Part print with two shaded views. Sizes in mm from the minimum x, y, z corner. A direction names the side the tool comes from. Round coordinates to 2 decimals unless told otherwise and drop trailing zeros. Loops run counter-clockwise (first coordinate to the right, second up) from the corner with the lowest first, then second, coordinate; pieces in that order, holes last. Notation, with made-up numbers: M -39.5,-1.5 L 8.5,-1.5 A11 ccw 8.5,17.5 Z; hole C 76.5,56.5 d1. An arc over 180 degrees is marked long. Use a Markdown table: item, result. Add a question column.
Item 1: Saw through at B-B on z = 45. Write the cut outline in (x, y), then the cut area to 3 significant figures.
Item 2: Tool access for the marked faces 1 and 2: list every direction of +Z, -Z, +X, -X, +Y, -Y with a clear straight run to the whole face (end or side of a thin tool).
Item 3: Saw through at C-C on y = 25. Write the cut outline in (x, z), then the cut area to 3 significant figures.
Item 4: Pin check, flat tips, straight feed: P1, Ø1, axis at x = 143, z = 96.5, coming from the +Y side; P2, Ø4, axis at y = 72, z = 77.5, coming from the -X side. Stop position of each tip, or through.
Item 5: Two-plate mould, pull along Z, no slides. Class the marked faces 3, 4, 5 and 6: +Z half, -Z half, draft (parallel to the pull), parting line (faces both ways), or undercut.
Item 6: Saw through at A-A on y = 7. Write the cut outline in (x, z).
Item 7: Saw through at D-D on x = 101.5. Write the cut outline in (y, z), then the cut area to 4 significant figures.
Item 8: Wall check: L1, parallel to X at y = 8, z = 79.5; L2, parallel to Z at x = 152, y = 27.5; L3, parallel to Y at x = 141, z = 103. Give the ranges that are in metal, low to high. Write a range as from..to.
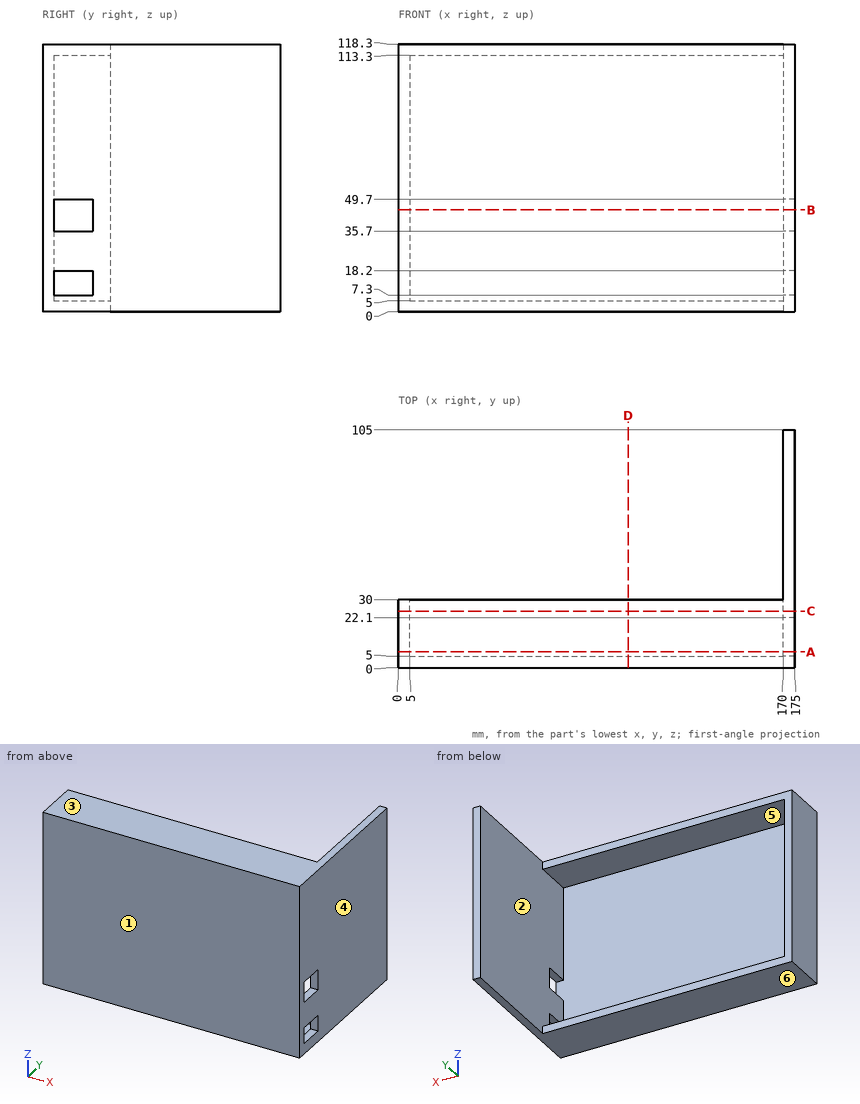
Entries:
| question | item | result |
|---|---|---|
| 1 | outline | M 0,0 L 175,0 L 175,5 L 5,5 L 5,30 L 0,30 Z; M 170,22.1 L 175,22.1 L 175,105 L 170,105 Z |
| 1 | area | 1,410 mm2 |
| 2 | face 1 | +Z, -Z, +X, -X, -Y |
| 2 | face 2 | +Y |
| 3 | outline | M 0,0 L 175,0 L 175,118.3 L 0,118.3 Z; hole M 5,5 L 170,5 L 170,113.3 L 5,113.3 Z |
| 3 | area | 2,830 mm2 |
| 4 | P1 | y = 5 |
| 4 | P2 | x = 170 |
| 5 | face 3 | +Z half |
| 5 | face 4 | draft |
| 5 | face 5 | undercut |
| 5 | face 6 | -Z half |
| 6 | outline | M 0,0 L 175,0 L 175,7.3 L 170,7.3 L 170,5 L 5,5 L 5,113.3 L 170,113.3 L 170,49.7 L 175,49.7 L 175,118.3 L 0,118.3 Z; M 170,18.2 L 175,18.2 L 175,35.7 L 170,35.7 Z |
| 7 | outline | M 0,0 L 30,0 L 30,5 L 5,5 L 5,113.3 L 30,113.3 L 30,118.3 L 0,118.3 Z |
| 7 | area | 841.5 mm2 |
| 8 | L1 | 0..5, 170..175 |
| 8 | L2 | 0..5, 113.3..118.3 |
| 8 | L3 | 0..5 |
